```python
from build123d import *

# Parameters (mm, degrees)
SKETCH1_W               = 20
SKETCH1_H               = 50
BOSS_EXTRUDE1_DEPTH     = 12
CUT_EXTRUDE1_REACH      = 54.383
SKETCH4_W               = 50
SKETCH4_H               = 9.5
BOSS_EXTRUDE2_DEPTH     = 8
SKETCH5_W               = 50
SKETCH5_H               = 9.5
BOSS_EXTRUDE3_DEPTH     = 8
CUT_EXTRUDE4_DEPTH      = 33.23740064
CUT_EXTRUDE4_DEPTH_BACK = 33.23740064
SKETCH10_R              = 2.75
SKETCH13_W              = 36
SKETCH13_H              = 50
CUT_EXTRUDE6_DEPTH      = 5.5
CUT_EXTRUDE7_REACH      = 33.064
SKETCH14_R              = 5.05


with BuildPart() as part:
    # Sketch1 → Boss-Extrude1 (new body)
    with BuildSketch(Plane(origin=(0, 0, 0), x_dir=(1, 0, 0), z_dir=(0, 1, 0))):
        Rectangle(SKETCH1_W, SKETCH1_H)
    extrude(amount=BOSS_EXTRUDE1_DEPTH)

    # Sketch2 → Cut-Extrude1 (cut, up to next)
    with BuildSketch(Plane.XY.offset(25), mode=Mode.PRIVATE) as cut_extrude1_sk1:
        Polygon((0, 9.5), (7.25, 9.5), (6.25, 12), (0, 12), (-6.25, 12), (-7.25, 9.5), align=None)
    cut_extrude1_tool1 = extrude(cut_extrude1_sk1.sketch, amount=-CUT_EXTRUDE1_REACH, mode=Mode.PRIVATE) & part.part
    add(cut_extrude1_tool1.solids().sort_by_distance((0, 10.719136, 25))[0], mode=Mode.SUBTRACT)

    # Sketch4 → Boss-Extrude2 (add)
    with BuildSketch(Plane.ZY.offset(10)):
        with Locations((0, 4.75)):
            Rectangle(SKETCH4_W, SKETCH4_H)
    extrude(amount=BOSS_EXTRUDE2_DEPTH)

    # Sketch5 → Boss-Extrude3 (add)
    with BuildSketch(Plane(origin=(10, 0, 0), x_dir=(0, 0, -1), z_dir=(1, 0, 0))):
        with Locations((0, 4.75)):
            Rectangle(SKETCH5_W, SKETCH5_H)
    extrude(amount=BOSS_EXTRUDE3_DEPTH)

    # Sketch10 → Cut-Extrude4 (cut, two sides: drawn at the far end of the back side and taken through both)
    with BuildSketch(Plane(origin=(0, 9.5, 0), x_dir=(1, 0, 0), z_dir=(0, 1, 0)).offset(-CUT_EXTRUDE4_DEPTH_BACK)):
        with Locations(Location((-12.5, 12.5, 0), (0, 0, 270))):
            Circle(SKETCH10_R)
        with Locations(Location((12.5, 12.5, 0), (0, 0, 270))):
            Circle(SKETCH10_R)
        with Locations(Location((-12.5, -12.5, 0), (0, 0, 270))):
            Circle(SKETCH10_R)
        with Locations(Location((12.5, -12.5, 0), (0, 0, 270))):
            Circle(SKETCH10_R)
    extrude(amount=CUT_EXTRUDE4_DEPTH + CUT_EXTRUDE4_DEPTH_BACK, mode=Mode.SUBTRACT)

    # Sketch13 → Cut-Extrude6 (cut)
    with BuildSketch(Plane.XZ):
        Rectangle(SKETCH13_W, SKETCH13_H)
    extrude(amount=-CUT_EXTRUDE6_DEPTH, mode=Mode.SUBTRACT)

    # Sketch14 → Cut-Extrude7 (cut, up to next)
    with BuildSketch(Plane(origin=(0, 9.5, 0), x_dir=(1, 0, 0), z_dir=(0, 1, 0)), mode=Mode.PRIVATE) as cut_extrude7_sk1:
        with Locations((-12.5, 12.5)):
            Circle(SKETCH14_R)
    cut_extrude7_tool1 = extrude(cut_extrude7_sk1.sketch, amount=CUT_EXTRUDE7_REACH, mode=Mode.PRIVATE) & part.part
    # Sketch14 → Cut-Extrude7 (cut, up to next)
    with BuildSketch(Plane(origin=(0, 9.5, 0), x_dir=(1, 0, 0), z_dir=(0, 1, 0)), mode=Mode.PRIVATE) as cut_extrude7_sk2:
        with Locations((12.5, 12.5)):
            Circle(SKETCH14_R)
    cut_extrude7_tool2 = extrude(cut_extrude7_sk2.sketch, amount=CUT_EXTRUDE7_REACH, mode=Mode.PRIVATE) & part.part
    # Sketch14 → Cut-Extrude7 (cut, up to next)
    with BuildSketch(Plane(origin=(0, 9.5, 0), x_dir=(1, 0, 0), z_dir=(0, 1, 0)), mode=Mode.PRIVATE) as cut_extrude7_sk3:
        with Locations((-12.5, -12.5)):
            Circle(SKETCH14_R)
    cut_extrude7_tool3 = extrude(cut_extrude7_sk3.sketch, amount=CUT_EXTRUDE7_REACH, mode=Mode.PRIVATE) & part.part
    # Sketch14 → Cut-Extrude7 (cut, up to next)
    with BuildSketch(Plane(origin=(0, 9.5, 0), x_dir=(1, 0, 0), z_dir=(0, 1, 0)), mode=Mode.PRIVATE) as cut_extrude7_sk4:
        with Locations((12.5, -12.5)):
            Circle(SKETCH14_R)
    cut_extrude7_tool4 = extrude(cut_extrude7_sk4.sketch, amount=CUT_EXTRUDE7_REACH, mode=Mode.PRIVATE) & part.part
    add(cut_extrude7_tool1.solids().sort_by_distance((-12.5, 9.5, -12.5))[0], mode=Mode.SUBTRACT)
    add(cut_extrude7_tool2.solids().sort_by_distance((12.5, 9.5, -12.5))[0], mode=Mode.SUBTRACT)
    add(cut_extrude7_tool3.solids().sort_by_distance((-12.5, 9.5, 12.5))[0], mode=Mode.SUBTRACT)
    add(cut_extrude7_tool4.solids().sort_by_distance((12.5, 9.5, 12.5))[0], mode=Mode.SUBTRACT)


solid = part.part
```
The listing builds one solid part. Answer for the finished solid, in the listing's coordinates (mm). A direction names the side the tool comes from. Coordinates: 2 decimals unless noted, no trailing zeros. Loops run counter-clockwise (first coordinate to the right, second up) from the corner with the lowest first, then second, coordinate; pieces in that order, holes last. Notation, with made-up numbers: M 86.25,-22.5 L 141.25,-22.5 A14 cw 141.25,-5.5 Z; hole C 40.25,39 d10. An arc over 180 degrees is marked long. Answer as CSV lines item,"result". Start each with the question number.
(1) The part is cut by section B-B (y = 11). Give the vertices of the cut face in (x, z), and give its area (3 significant figures).
(2) The part is cut by section C-C (z = -12.5). Give the vertices of the cut face in (x, y), and give its area (4 significant figures).
(3) The part is cut by section A-A (x = -12.5). Give the vertices of the cut face in (y, z).
(4) The mould has two halves that part along X. Classify faces 5 (the flat face through (10, 11, 0)), 6 (the flat face through (14, 9.5, 0)), 7 (the cylindrical face through (-10.18, 7.47, 13.98)): pulls with the +X half, pulls with the -X half, needs draft (parallel to the pull), parting line crosses it, or undercut.
(5) The part is cut by section D-D (y = 7). Give the vertices of the cut face in (x, z), and give its area (3 significant figures).
(6) For faces 1 (the cylindrical face through (7.45, 10.73, -12.57)), 2 (the flat face through (10, 11, -21)), 3 (the flat face through (6.76, 10.73, 0.35)), 4 (the flat face through (-10, 11, -21)), determine the directions among +Z, -Z, +X, -X, +Y, -Y from which every point of the face is accessible in a straight line to the end or side of a thin tool.
(7) Find the intervals of material crossed by L1, parallel to Z at x = -12.5, y = 7.25; L2, parallel to X at y = 7.4, z = -12.5; L3, parallel to X at y = 9, z = 13.5, in increasing order. Write a range as [from, to].
(8) Given pin 1 (0.8 mm diameter, centred on y = 10.5, z = 3, fed in from -X); pin 2 (1 mm diameter, centred on x = 3.5, z = 10, fed in from +Y); pin 3 (2 mm diameter, centred on y = 11, z = 3, fed in from +X), each flat-ended and moving along its own axis, determine where each tip first touches the part or whether it passes through.
Determined:
1,outline,"M -10,-25 L -6.65,-25 L -6.65,25 L -10,25 L -10,16.89 A5.05 cw -10,8.11 L -10,-8.11 A5.05 cw -10,-16.89 Z; M 6.65,-25 L 10,-25 L 10,-16.89 A5.05 cw 10,-8.11 L 10,8.11 A5.05 cw 10,16.89 L 10,25 L 6.65,25 Z"
1,area,"271 mm2"
2,outline,"M -18,5.5 L -15.25,5.5 L -15.25,9.5 L -18,9.5 Z; M -9.75,5.5 L 9.75,5.5 L 9.75,9.5 L 7.45,9.5 L 7.45,12 L 6.25,12 L 7.25,9.5 L -7.25,9.5 L -6.25,12 L -7.45,12 L -7.45,9.5 L -9.75,9.5 Z; M 15.25,5.5 L 18,5.5 L 18,9.5 L 15.25,9.5 Z"
2,area,"103.5 mm2"
3,outline,"M 5.5,-25 L 9.5,-25 L 9.5,-15.25 L 5.5,-15.25 Z; M 5.5,-9.75 L 9.5,-9.75 L 9.5,9.75 L 5.5,9.75 Z; M 5.5,15.25 L 9.5,15.25 L 9.5,25 L 5.5,25 Z"
4,face 5,"pulls with the +X half"
4,face 6,"needs draft"
4,face 7,"undercut"
5,outline,"M -18,-25 L 18,-25 L 18,25 L -18,25 Z; hole C -12.5,-12.5 d5.5; hole C -12.5,12.5 d5.5; hole C 12.5,-12.5 d5.5; hole C 12.5,12.5 d5.5"
5,area,"1,700 mm2"
6,face 1,"+X, +Y"
6,face 2,"+Z, -Z, +X, +Y"
6,face 3,"+Z, -Z"
6,face 4,"+Z, -Z, -X, +Y"
7,L1,"[-25, -15.25], [-9.75, 9.75], [15.25, 25]"
7,L2,"[-18, -15.25], [-9.75, 9.75], [15.25, 18]"
7,L3,"[-18, -15.06], [-9.94, 9.94], [15.06, 18]"
8,pin 1,"x = -10"
8,pin 2,"y = 9.5"
8,pin 3,"x = 10"
